Verification items for this drawing (mm, ordinates from the low corner). A direction names the side the tool comes from. Give positions to 0.01 mm unless a question says otherwise; leave off trailing zeros. Loops run counter-clockwise (first coordinate to the right, second up) from the corner with the lowest first, then second, coordinate; pieces in that order, holes last. Notation, with made-up numbers: M 43,41 L 80,41 A31 cw 80,74 Z; hole C 23.25,-17.75 d10. An arc over 180 degrees is marked long. Answer in a Markdown table with one row per item.
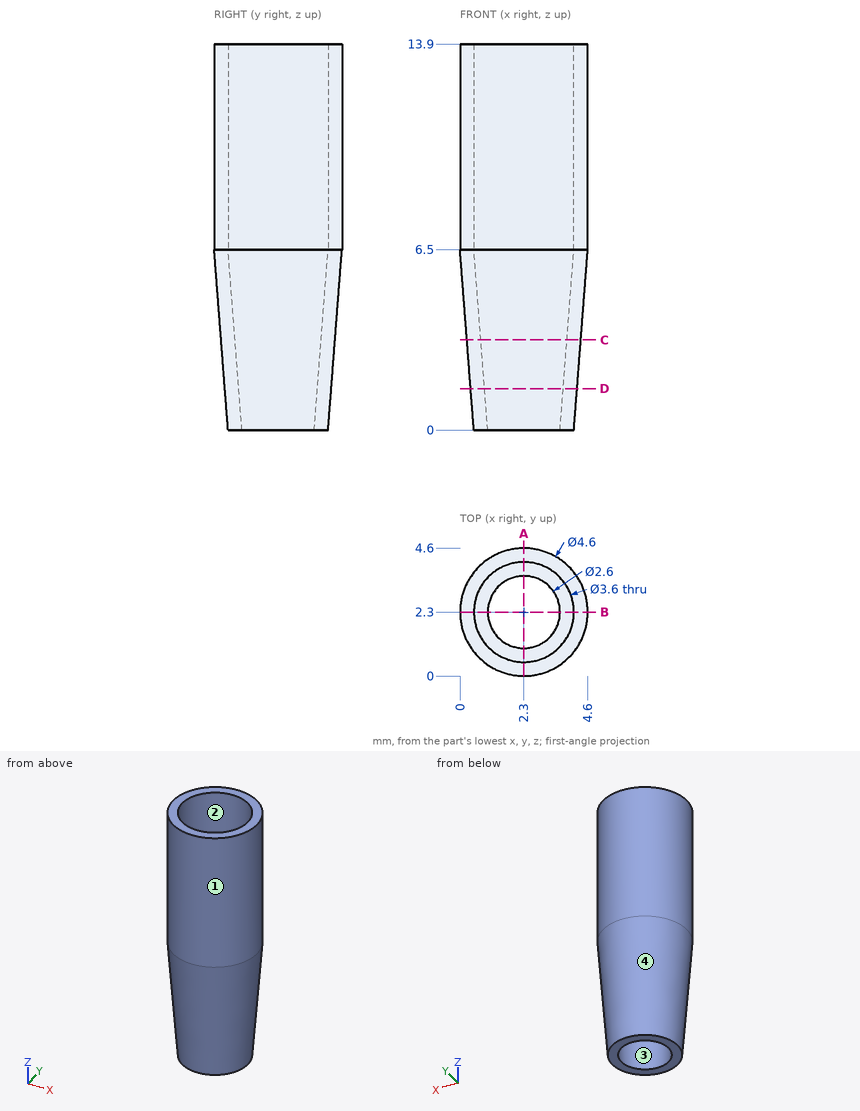
Item 1: Sectioned sample at A-A (x = 2.3). Record the cut outline in (y, z).
Reported:
| item | result |
|---|---|
| outline | M 0,6.5 L 0.5,0 L 1,0 L 0.5,6.5 L 0.5,13.9 L 0,13.9 Z; M 3.6,0 L 4.1,0 L 4.6,6.5 L 4.6,13.9 L 4.1,13.9 L 4.1,6.5 Z |
Item 2: Sectioned sample at D-D (z = 1.5). Record the cut outline in (x, y), and give its area (3 significant figures).
Reported:
| item | result |
|---|---|
| outline | C 2.3,2.3 d3.83; hole C 2.3,2.3 d2.83 |
| area | 5.23 mm^2 |
Item 3: Release check for a two-part mould opening along Y. For the marked faces 3 and 4 record: released by +Y, released by -Y, zero draft, split by the parting line, or undercut.
Reported:
| item | result |
|---|---|
| face 3 | undercut |
| face 4 | split by the parting line |
Item 4: Tool access check on the marked faces 1 and 2. Record the directions out of +Z, -Z, +X, -X, +Y, -Y that give a thin tool (end or side, any length) a straight path to the whole face; none if there is none.
Reported:
| item | result |
|---|---|
| face 1 | +Z, -Z |
| face 2 | +Z |
Item 5: Sectioned sample at C-C (z = 3.25). Record the cut outline in (x, y), and give its area (3 significant figures).
Reported:
| item | result |
|---|---|
| outline | C 2.3,2.3 d4.1; hole C 2.3,2.3 d3.1 |
| area | 5.65 mm^2 |
Item 6: Go/stop test with flat-tipped pins: pin 1 (2 mm diameter, centred on y = 1, z = 10, fed in from -X); pin 2 (1 mm diameter, centred on x = 3, z = 10.5, fed in from +Y). Record where each tip stops, or that it passes through.
Reported:
| item | result |
|---|---|
| pin 1 | stops at x = 0.02 |
| pin 2 | stops at y = 4.59 |
Item 7: Scan lines: L1, parallel to Y at x = 2.3, z = 11.25; L2, parallel to X at y = 0.9, z = 4.75; L3, parallel to Y at x = 1.2, z = 4.25. Record each from-to range of solid material in increasing order. Write a range as [from, to].
Reported:
| item | result |
|---|---|
| L1 | y = [0, 0.5], [4.1, 4.6] |
| L2 | x = [0.65, 1.4], [3.2, 3.95] |
| L3 | y = [0.48, 1.1], [3.5, 4.12] |
